Here's how the part is built. I have some questions about the finished solid (model axes, mm). Round coordinates to 2 decimals unless told otherwise and drop trailing zeros. Order: outer loops, then holes, each group sorted by start corner. A loop starts at its lowest first (then second) coordinate and runs counter-clockwise, first axis right, second up.
Autodesk Inventor part; units mm, degrees
ref_plane "YZ Plane" through (0, 0, 0) normal (1, 0, 0) x (0, 1, 0)
ref_plane "XZ Plane" through (0, 0, 0) normal (0, 1, 0) x (-1, 0, 0)
ref_plane "XY Plane" through (0, 0, 0) normal (0, 0, 1) x (1, 0, 0)
sketch "Sketch1" plane through (0, 0, 0) normal (0, 1, 0) x (-1, 0, 0)
  line L0 (5.7735, 0) -> (-7.7265, 23.3827)
  line L1 (-7.7265, 23.3827) -> (-6.6962, 15.9904)
  line L2 (-6.6962, 15.9904) -> (-7.5, 12.9904)
  line L3 (-7.5, 12.9904) -> (0, 0)
  line L4 (0, 0) -> (-7.5, -12.9904)
  line L5 (-7.5, -12.9904) -> (-6.6962, -15.9904)
  line L6 (-6.6962, -15.9904) -> (-7.7265, -23.3827)
  line L7 (-7.7265, -23.3827) -> (5.7735, 0)
  line L8 (14.7308, 0) -> (-3.2807, 0) construction
  dimension "d0" = 0
  dimension "d1" = 0
  dimension "d2" = 0
  dimension "d3" = 60
  dimension "d4" = 60
  dimension "d5" = 5
  dimension "d6" = 135
  dimension "d7" = 135
  dimension "d8" = 15
  dimension "d9" = 15
  dimension "d10" = 3
  dimension "d11" = 3
  dimension "d12" = 27
  dimension "d13" = 27
extrude "Extrusion1" add sketch "Sketch1" along normal blind 3
chamfer "Chamfer1" distance 1.5 angle 45 6 edges at (3.75, 3, 6.4952) (3.75, 3, -6.4952) (7.0981, 3, -14.4904) (7.0981, 3, 14.4904) (7.2113, 3, 19.6865) (7.2113, 3, -19.6865)
chamfer "Chamfer2" distance 1.5 angle 45 2 edges at (-0.0217, 3, 9.9623) (-0.0217, 3, -9.9623)
chamfer "Chamfer3" distance 1.5 angle 45 6 edges at (3.75, 0, -6.4952) (7.0981, 0, -14.4904) (7.2113, 0, -19.6865) (3.75, 0, 6.4952) (7.2113, 0, 19.6865) (7.0981, 0, 14.4904)
chamfer "Chamfer4" distance 1.5 angle 45 2 edges at (-0.0214, 0, -9.9629) (-0.0214, 0, 9.9629)
properties part number "SpeedRank"
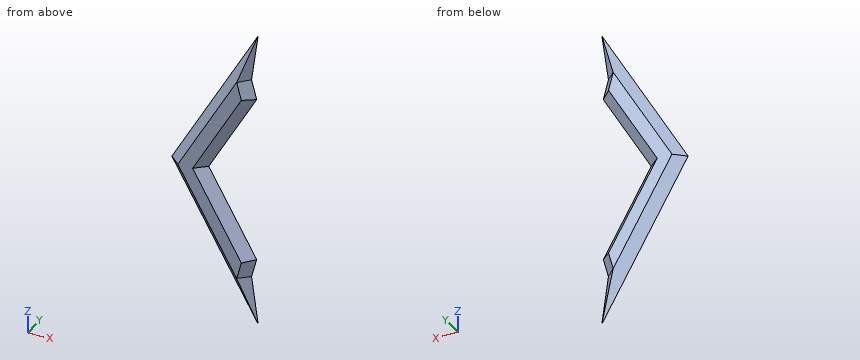
1. I need wall thicknesses on probe 1 along Z at (x, y) = (2.5, 1.85); probe 2 along Z at (x, y) = (0.75, 1.3); probe 3 along X at (y, z) = (0.7, -13). Which ranges of each line are inside material? Lowest first, please.
Evaluation:
probe 1: z = -13.63 to -5.03, 5.03 to 13.63
probe 2: z = -10.9 to -1.7, 1.7 to 10.9
probe 3: x = 2.66 to 6.58
2. If we section it at B-B, the plane y = 0.75: Write out the boundary of the cut face in (x, z).
Evaluation:
outline: (-4.91, 0) - (6.45, -19.68) - (5.93, -15.94) - (6.7, -13.1) - (-0.87, 0) - (6.7, 13.1) - (5.93, 15.94) - (6.45, 19.68) - close
3. I'm going to push flat-ended pins straight in: P1, Ø1.5, axis at x = -0.5, y = 2, coming from the -Z side; P2, Ø1.5, axis at x = 2, y = 1, coming from the -Z side; P3, Ø5, axis at x = 3.5, z = -18, coming from the -Y side. Where does each tip first touch, or does it pass through?
Evaluation:
P1: stops at z = -10.1
P2: stops at z = -14.43
P3: stops at y = 0.05
